Autodesk Inventor part; units mm, degrees
ref_plane "YZ Plane" through (0, 0, 0) normal (1, 0, 0) x (0, 1, 0)
ref_plane "XZ Plane" through (0, 0, 0) normal (0, 1, 0) x (-1, 0, 0)
ref_plane "XY Plane" through (0, 0, 0) normal (0, 0, 1) x (1, 0, 0)
sketch "Sketch3" plane through (0, 0, 0) normal (0, 1, 0) x (-1, 0, 0)
  circle A0 centre (0, 0) radius 12.7
  circle A1 centre (0, 0) radius 19.05
  dimension "d7" = 25.4
  dimension "d8" = 38.1
extrude "Extrusion1" add sketch "Sketch3" along normal mid plane 25.4
chamfer "Chamfer1" distance 3.175 angle 45 1 edges at (12.7, 12.7, 0)
properties part number "Tube"
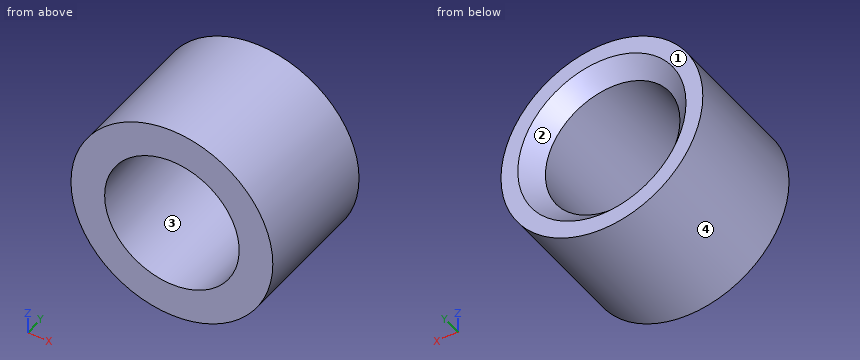
The model under review builds one solid part; all positions refer to its coordinate system, in mm. Face numbers are marked on the shaded views. Round coordinates to 2 decimals unless told otherwise and drop trailing zeros. Order: outer loops, then holes, each group sorted by start corner. A loop starts at its lowest first (then second) coordinate and runs counter-clockwise, first axis right, second up. Notation, with made-up numbers: (40, 72.25) - (69, 72.25) arc R12 cw to (69, 83.25) - close; hole circle Ø10 at (-7, 49.25). An arc over 180 degrees is marked (long way). Answer in a Markdown table with one row per item.
(1) Take a section at A-A on z = 0. Write out the cut boundary in (x, y) (3 decimals), plus the area to 4 significant figures.
Result set:
| item | result |
|---|---|
| outline | (-19.05, -12.7) - (-12.7, -12.7) - (-12.7, 9.525) - (-15.875, 12.7) - (-19.05, 12.7) - close; (12.7, -12.7) - (19.05, -12.7) - (19.05, 12.7) - (15.875, 12.7) - (12.7, 9.525) - close |
| area | 312.5 mm2 |
(2) For line 1 (Z direction, x = 0, y = -0.25); line 2 (Z direction, x = 2, y = 10.75); line 3 (X direction, y = 4, z = 8.5), list the stretches that pass through material, from the lowest coordinate up. Write a range as from..to.
Result set:
| item | result |
|---|---|
| line 1 | z = -19.05..-12.7, 12.7..19.05 |
| line 2 | z = -18.94..-13.78, 13.78..18.94 |
| line 3 | x = -17.05..-9.44, 9.44..17.05 |
(3) Take a section at C-C on y = 1. Write out the cut boundary in (x, z).
Result set:
| item | result |
|---|---|
| outline | circle Ø38.1 at (0, 0); hole circle Ø25.4 at (0, 0) |
(4) Clearance check with flat-ended pins moving along their axes: P1, Ø10, axis at x = 10, z = -0.5, coming from the +Y side; P2, Ø2, axis at x = -10, y = -9, coming from the -Z side; P3, Ø5, axis at y = 4.5, z = -12, coming from the -X side; P4, Ø2, axis at x = -15, z = 13.5, coming from the -Y side. State where each tip first meets the part, or that it passes through.
Result set:
| item | result |
|---|---|
| P1 | stops at y = 11.84 |
| P2 | stops at z = -16.79 |
| P3 | stops at x = -16.51 |
| P4 | passes through |
(5) Mouldability with a two-part tool opening along X and no side actions: class the marked faces 1, 2, 3 and 4 as released by +X, released by -X, zero draft, split by the parting line, or undercut.
Result set:
| item | result |
|---|---|
| face 1 | zero draft |
| face 2 | undercut |
| face 3 | undercut |
| face 4 | split by the parting line |
(6) Take a section at B-B on x = 0. Write out the cut boundary in (y, z) (3 decimals).
Result set:
| item | result |
|---|---|
| outline | (-12.7, -19.05) - (12.7, -19.05) - (12.7, -15.875) - (9.525, -12.7) - (-12.7, -12.7) - close; (-12.7, 12.7) - (9.525, 12.7) - (12.7, 15.875) - (12.7, 19.05) - (-12.7, 19.05) - close |
